Read the model definition and answer for the solid it produces. Units are mm, in the model's axes. Face numbers are marked on the shaded views. A direction names the side the tool comes from. Coordinates: 2 decimals unless noted, no trailing zeros. Order: outer loops, then holes, each group sorted by start corner. A loop starts at its lowest first (then second) coordinate and runs counter-clockwise, first axis right, second up. Notation, with made-up numbers: (65, 83) -> (69, 83) arc R27 ccw to (69, 102) -> close; hole circle Ø10 at (61, 29). An arc over 180 degrees is marked (long way). Answer in a Markdown table with one row per item.
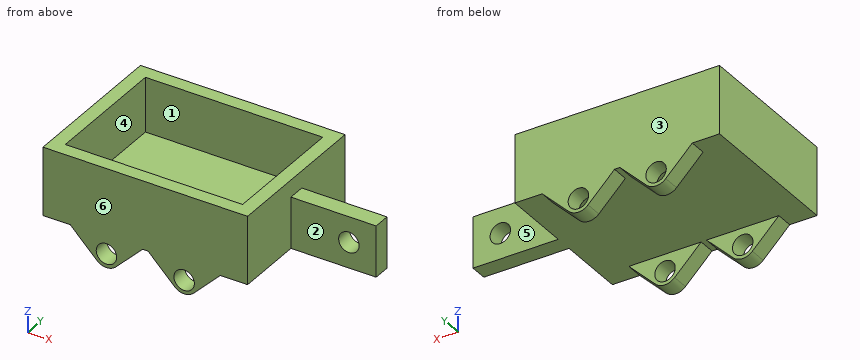
from build123d import *

# Parameters (mm, degrees)
F0_W      = 76.2
F0_H      = 57.15
F1_DEPTH  = 25.4
F2_T      = -5.08
F4_DEPTH  = 6.35
F5_R      = 5.08
F8_DEPTH  = 6.35
F9_D      = 7.62
F10_R     = 5.08
F11_W     = 6.35
F11_H     = 19.05
F12_DEPTH = 31.75
F14_D     = 7.62


with BuildPart() as f1:
    # F0 (on Top) → F1 (new body)
    with BuildSketch(Plane.XY):
        Rectangle(F0_W, F0_H)
    extrude(amount=F1_DEPTH)

    # F2
    f2_openings = [f1.faces().sort_by_distance(p)[0] for p in [
        (0, 0, 25.4),
    ]]
    offset(amount=F2_T, openings=f2_openings)

    # F3 (on face) → F4 (join)
    with BuildSketch(Plane.XZ.offset(28.575)):
        Polygon((-0.9992316368, 0), (-27.94, 0), (-14.4696158184, -13.4703841816), align=None)
        Polygon((27.94, 0), (0.9992316368, 0), (14.4696158184, -13.4703841816), align=None)
    extrude(amount=-F4_DEPTH)

    # F5
    f5_edges = [f1.edges().sort_by_distance(p)[0] for p in [
        (-14.469616, -25.4, -13.470384),
        (14.469616, -25.4, -13.470384),
    ]]
    fillet(f5_edges, radius=F5_R)

    # F7 (on face) → F8 (join)
    with BuildSketch(Plane(origin=(0, 28.575, 0), x_dir=(-1, 0, 0), z_dir=(0, 1, 0))):
        Polygon((-0.9992316368, 0), (-27.94, 0), (-14.4696158184, -13.4703841816), align=None)
        Polygon((27.94, 0), (0.9992316368, 0), (14.4696158184, -13.4703841816), align=None)
    extrude(amount=-F8_DEPTH)

    # F9 (through all)
    with Locations(Plane.XZ.offset(28.575)):
        with Locations((-14.4696158184, -6.2861792847), (14.4696158184, -6.2861792847)):
            Hole(F9_D / 2)

    # F10
    f10_edges = [f1.edges().sort_by_distance(p)[0] for p in [
        (14.469616, 25.4, -13.470384),
        (-14.469616, 25.4, -13.470384),
    ]]
    fillet(f10_edges, radius=F10_R)

    # F11 (on face) → F12 (join)
    with BuildSketch(Plane.YZ.offset(38.1)):
        with Locations((0, 9.525)):
            Rectangle(F11_W, F11_H)
    extrude(amount=F12_DEPTH)

    # F14 (through all)
    with Locations(Plane(origin=(0, 3.175, 0), x_dir=(-1, 0, 0), z_dir=(0, 1, 0))):
        with Locations((-59.69, 9.525)):
            Hole(F14_D / 2)


solid = f1.part
Q1. The part is cut by section B-B (z = 8). Write down the section's boundary in (x, y) (3 decimals), then the cut area to 3 significant figures.
Outcome:
| item | result |
|---|---|
| outline | (-38.1, -28.575) -> (38.1, -28.575) -> (38.1, -3.175) -> (56.199, -3.175) -> (56.199, 3.175) -> (38.1, 3.175) -> (38.1, 28.575) -> (-38.1, 28.575) -> close; (63.181, -3.175) -> (69.85, -3.175) -> (69.85, 3.175) -> (63.181, 3.175) -> close; hole (-33.02, -23.495) -> (33.02, -23.495) -> (33.02, 23.495) -> (-33.02, 23.495) -> close |
| area | 1,410 mm² |
Q2. The part is cut by section D-D (y = 18.5). Write down the section's boundary in (x, z).
Outcome:
| item | result |
|---|---|
| outline | (-38.1, 0) -> (38.1, 0) -> (38.1, 25.4) -> (33.02, 25.4) -> (33.02, 5.08) -> (-33.02, 5.08) -> (-33.02, 25.4) -> (-38.1, 25.4) -> close |
Q3. Given pin 1 (4 mm diameter, centred on x = 3, z = -4.5, fed in from -Y) (3 decimals); pin 2 (1.9 mm diameter, centred on x = 49, y = 1.5, fed in from +Z); pin 3 (9 mm diameter, centred on x = 59.69, z = 9.525, fed in from +Y) (3 decimals); pin 4 (10 mm diameter, centred on y = -12.5, z = 14, fed in from +X), each flat-ended and moving along its own axis, determine where each tip first touches the part or whether it passes through.
Outcome:
| item | result |
|---|---|
| pin 1 | y = -28.575 |
| pin 2 | z = 19.05 |
| pin 3 | y = 3.175 |
| pin 4 | x = 38.1 |
Q4. The part is cut by section C-C (z = 22.5). Write down the section's boundary in (x, y) (3 decimals), then the cut area to 3 significant figures.
Outcome:
| item | result |
|---|---|
| outline | (-38.1, -28.575) -> (38.1, -28.575) -> (38.1, 28.575) -> (-38.1, 28.575) -> close; hole (-33.02, -23.495) -> (33.02, -23.495) -> (33.02, 23.495) -> (-33.02, 23.495) -> close |
| area | 1,250 mm² |
Q5. For a pull along Y with two mould halves and no side action, classify the marked faces 4, 5 and 6 as pulls with the +Y half, pulls with the -Y half, needs draft (parallel to the pull), parting line crosses it, or undercut.
Outcome:
| item | result |
|---|---|
| face 4 | undercut |
| face 5 | pulls with the +Y half |
| face 6 | pulls with the -Y half |
Q6. The part is cut by section A-A (x = 59.69). Write down the section's boundary in (y, z) (3 decimals).
Outcome:
| item | result |
|---|---|
| outline | (-3.175, 0) -> (3.175, 0) -> (3.175, 5.715) -> (-3.175, 5.715) -> close; (-3.175, 13.335) -> (3.175, 13.335) -> (3.175, 19.05) -> (-3.175, 19.05) -> close |
Q7. For the marked faces 1, 2 and 3, determine the directions among +Z, -Z, +X, -X, +Y, -Y from which every point of the face is accessible in a straight line to the end or side of a thin tool.
Outcome:
| item | result |
|---|---|
| face 1 | +Z |
| face 2 | +Z, -Z, +X, -Y |
| face 3 | +Z, -Z, +X, -X, +Y |
Q8. Consider line 1 (Y direction, x = -13, z = 22) (3 decimals); line 2 (X direction, y = -21, z = 7); line 3 (Z direction, x = 59.69, y = 0) (3 decimals). Determine where each line is inside the solid, lowest interval first.
Outcome:
| item | result |
|---|---|
| line 1 | -28.575 to -23.495, 23.495 to 28.575 |
| line 2 | -38.1 to -33.02, 33.02 to 38.1 |
| line 3 | 0 to 5.715, 13.335 to 19.05 |
